Input: part model. Units: mm. Frame: model coordinates. A direction names the side the tool comes from. Give positions to 0.01 mm unless a question says otherwise; leave off trailing zeros. Loops run counter-clockwise (first coordinate to the right, second up) from the corner with the lowest first, then second, coordinate; pieces in that order, holes last. Notation, with made-up numbers: (82.25, 54.5) - (129.25, 54.5) arc R22 cw to (129.25, 88.5) - close; hole circle Ø9 at (-24, 41). An arc over 180 degrees is marked (long way). One line per item, written item: value.
from build123d import *

# Parameters (mm, degrees)
BOSS_EXTRUDE1_DEPTH                              = 38.1
SKETCH3_W                                        = 20.066
SKETCH3_H                                        = 28.2194
CUT_EXTRUDE1_DEPTH                               = 1.021241984
CUT_EXTRUDE1_DEPTH_BACK                          = 40.5224
F_10_24_TAPPED_HOLE1_D                           = 3.7973
F_10_24_TAPPED_HOLE1_DEPTH                       = 12.954
F_10_24_TAPPED_HOLE1_TIP                         = 1.140824014
CBORE_FOR_1_4_SOCKET_SHOULDER_SCREW1_D           = 6.3754
CBORE_FOR_1_4_SOCKET_SHOULDER_SCREW1_DEPTH       = 9.017
CBORE_FOR_1_4_SOCKET_SHOULDER_SCREW1_CBORE_D     = 10.2616
CBORE_FOR_1_4_SOCKET_SHOULDER_SCREW1_CBORE_DEPTH = 3.8862
SKETCH13_R                                       = 3.4925
CUT_EXTRUDE2_DEPTH                               = 38.322374195
FILLET1_R                                        = 6.35


with BuildPart() as part:
    # Sketch1 → Boss-Extrude1 (new body)
    with BuildSketch(Plane.XY):
        with BuildLine():
            Line((-19.7612, 0), (19.7612, 0))
            Line((19.7612, 0), (19.7612, 8.89))
            Line((19.7612, 8.89), (17.037205242, 8.89))
            ThreePointArc((17.037205242, 8.89), (1.975351394, 15.011688564), (-4.545142708, 29.905233101))
            ThreePointArc((-4.545142708, 29.905233101), (-12.548269927, 37.3126), (-19.7612, 29.1338))
            Line((-19.7612, 29.1338), (-19.7612, 0))
        make_face()
    extrude(amount=-BOSS_EXTRUDE1_DEPTH)

    # Sketch3 → Cut-Extrude1 (cut, two sides)
    with BuildSketch(Plane.ZY.offset(19.7612)) as cut_extrude1_sk:
        with Locations((-19.05, 23.212674195)):
            Rectangle(SKETCH3_W, SKETCH3_H)
    extrude(amount=CUT_EXTRUDE1_DEPTH, mode=Mode.SUBTRACT)
    extrude(cut_extrude1_sk.sketch, amount=-CUT_EXTRUDE1_DEPTH_BACK, mode=Mode.SUBTRACT)

    # #10-24 Tapped Hole1
    with Locations(Plane.XY):
        with Locations((-12.162441984, 29.702374195)):
            Hole(F_10_24_TAPPED_HOLE1_D / 2, depth=F_10_24_TAPPED_HOLE1_DEPTH)
            with Locations((0, 0, -(F_10_24_TAPPED_HOLE1_DEPTH + F_10_24_TAPPED_HOLE1_TIP / 2))):  # 118° drill point
                Cone(0, F_10_24_TAPPED_HOLE1_D / 2, F_10_24_TAPPED_HOLE1_TIP, mode=Mode.SUBTRACT)

    # CBORE for 1/4 Socket Shoulder Screw1
    with Locations(Plane(origin=(0, 0, -38.1), x_dir=(-1, 0, 0), z_dir=(0, 0, -1))):
        with Locations((12.162441984, 29.702374195)):
            CounterBoreHole(CBORE_FOR_1_4_SOCKET_SHOULDER_SCREW1_D / 2, CBORE_FOR_1_4_SOCKET_SHOULDER_SCREW1_CBORE_D / 2, CBORE_FOR_1_4_SOCKET_SHOULDER_SCREW1_CBORE_DEPTH, depth=CBORE_FOR_1_4_SOCKET_SHOULDER_SCREW1_DEPTH)

    # Sketch13 → Cut-Extrude2 (cut, through all)
    with BuildSketch(Plane.XZ):
        with Locations((-12.0904, -19.05)):
            Circle(SKETCH13_R)
        with Locations((10.16, -19.05)):
            Circle(SKETCH13_R)
    extrude(amount=-CUT_EXTRUDE2_DEPTH, mode=Mode.SUBTRACT)

    # Fillet1
    fillet1_edges = [part.edges().sort_by_distance(p)[0] for p in [
        (19.7612, 4.445, -38.1),
        (19.7612, 4.445, 0),
    ]]
    fillet(fillet1_edges, radius=FILLET1_R)


solid = part.part
Item 1: Pin query (flat end, axial travel): P1, Ø1.5, axis at x = -0.5, z = -26, coming from the +Y side; P2, Ø8, axis at x = -12.16, y = 29.7, coming from the -Z side; P3, Ø1.5, axis at y = 8, z = -9, coming from the -X side. Return the tip coordinate at first contact, or that it passes through.
Verdict:
P1: stops at y = 9.1
P2: stops at z = -34.21
P3: stops at x = -19.76
Item 2: Access query for faces 1 (the face through (-7, 15, 0)), 2 (the face through (-11, 20, -9.017)), 3 (the face through (-11.05, 24.694, -36.184)). Directions: +Z, -Z, +X, -X, +Y, -Y. A direction counts if a zero-diameter tool reaches every point of the face in a straight line with its end or side. Return the directions, or none.
Verdict:
face 1: +Z, +X, -X, +Y, -Y
face 2: +X, -X, +Y
face 3: -Z
Item 3: Section C-C, the plane x = 10.16. Output: boundary loops of the cut face in (y, z).
Verdict:
outline: (0, -38.1) - (10.01, -38.1) - (10.01, -29.08) - (9.1, -29.08) - (9.1, -22.54) - (0, -22.54) - close; (0, -15.56) - (9.1, -15.56) - (9.1, -9.02) - (10.01, -9.02) - (10.01, 0) - (0, 0) - close
Item 4: Material intervals for L1, parallel to Z at x = -10, y = 9.5; L2, parallel to Z at x = -10.5, y = 26.5; L3, parallel to Y at x = 6, z = -28, sorted ascending.
Verdict:
L1: z = -38.1 to -29.08, -9.02 to 0
L2: z = -34.21 to -29.08, -9.02 to 0
L3: y = 0 to 9.1
Item 5: Section D-D, the plane y = 17.5. Output: boundary loops of the cut face in (x, z).
Verdict:
outline: (-19.76, -38.1) - (-0.22, -38.1) - (-0.22, -29.08) - (-19.76, -29.08) - close; (-19.76, -9.02) - (-0.22, -9.02) - (-0.22, 0) - (-19.76, 0) - close
Item 6: Section B-B, the plane y = 4. Count the separate pieces of the cut face and the enclosed holes in it, and give its area (3 significant figures).
Verdict:
separate pieces: 1
enclosed holes: 2
area: 1,410 mm^2
Item 7: Draft query along X for faces 4 (the face through (-19.761, 8, -19)), 5 (the face through (-10, 27, -34.214)), 6 (the face through (18, 8.89, -19)). Return one class per face: pulls with the +X half, pulls with the -X half, needs draft (parallel to the pull), parting line crosses it, or undercut.
Verdict:
face 4: pulls with the -X half
face 5: undercut
face 6: needs draft
Item 8: Section A-A, the plane z = -19.05. Output: boundary loops of the cut face in (x, y).
Verdict:
outline: (-19.76, 0) - (-15.58, 0) - (-15.58, 9.1) - (-19.76, 9.1) - close; (-8.6, 0) - (6.67, 0) - (6.67, 9.1) - (-8.6, 9.1) - close; (13.65, 0) - (19.76, 0) - (19.76, 8.89) - (17.04, 8.89) arc R21.59 cw to (14.01, 9.1) - (13.65, 9.1) - close
